Build history of the part. All positions in model axes, mm. A direction names the side the tool comes from. Give positions to 0.01 mm unless a question says otherwise; leave off trailing zeros. Order: outer loops, then holes, each group sorted by start corner. A loop starts at its lowest first (then second) coordinate and runs counter-clockwise, first axis right, second up. Notation, with made-up numbers: (-29.75, 66) - (-22.75, 66) arc R38 ccw to (-22.75, 105) - close; hole circle Ø11 at (-29, -18). An arc over 180 degrees is marked (long way). Write each question's results on one line, items separated by ' | '. Start each with the question number.
from build123d import *

# Parameters (mm, degrees)
SKETCH1_W                  = 127.078191072
SKETCH1_H                  = 113.282646321
BOSS_EXTRUDE1_DEPTH        = 39.624
SHELL_1_T                  = -2.54
OFFICIAL_RIB_BLOCK20_START = -2.54
OFFICIAL_RIB_BLOCK20_DEPTH = 2.54


with BuildPart() as part:
    # Sketch1 → Boss-Extrude1 (new body)
    with BuildSketch(Plane(origin=(0, 0, 0), x_dir=(1, 0, 0), z_dir=(0, 1, 0))):
        with Locations((1.06119575, 7.295720781)):
            Rectangle(SKETCH1_W, SKETCH1_H)
    extrude(amount=BOSS_EXTRUDE1_DEPTH)

    # 抽壳1
    shell_1_openings = [part.faces().sort_by_distance(p)[0] for p in [
        (1.06119575, 39.624, -7.295720782),
    ]]
    offset(amount=SHELL_1_T, openings=shell_1_openings, kind=Kind.INTERSECTION)

    # official_rib_block20: read off the stored shape, not the designer's step
    # official_rib_block20 outline → official_rib_block20 (add)
    with BuildSketch(Plane(origin=(0.729572078, 0, -0.729572078), x_dir=(0.7071067811865477, 0, 0.7071067811865475), z_dir=(-0.7071067811865475, 0, 0.7071067811865477)).offset(OFFICIAL_RIB_BLOCK20_START)):
        Polygon((-85.796761505, 21.08206499), (-85.796761505, 2.54), (69.764888407, 2.54), (69.764888407, 33.885045833), (7.726, 25.357), (-34.23, 35.134), align=None)
    extrude(amount=OFFICIAL_RIB_BLOCK20_DEPTH)


solid = part.part
Item 1: Which spindle directions (+Z, -Z, +X, -X, +Y, -Y) get a long thin tool onto all of the face, cutting with end or side? Do faces 1 (the flat face through (-3, 15.44, -8.05)), 2 (the flat face through (64.6, 20, -7)). Say none if no direction does.
Item 2: Cut at B-B, the plane z = -20.5. List the corners of the cut face in (x, y), then the cut area to 3 significant figures.
Item 3: Two-plate mould, pull along X, no slides. Class faces 3 (the flat face through (-62.478, 20, -7)), 4 (the flat face through (0, 0, -8)), 5 (the flat face through (15, 2.54, -20)): +X half, -X half, draft (parallel to the pull), parting line (faces both ways), or undercut.
Item 4: Flat gauge pins, fed straight in: pin 1 Ø8 at (x, z) = (8, -24) entering from +Y; pin 2 Ø10 at (x, z) = (-33, -41.5) entering from +Y. Where does each tip first touch, or does it go through?
Item 5: Probe line 1 along X through (y, z) = (33, -50); line 2 along Z through (x, y) = (23.5, 17); line 3 along X through (y, z) = (12, 40). List the from-to ranges inside material, lowest first. Write a range as from..to.
Item 6: Cut at A-A, the plane y = 8. List the corners of the cut face in (x, z).
Item 7: Cut at C-C, the plane x = -40. List the corners of the cut face in (y, z), then the cut area to 3 significant figures.
Values found:
1) face 1: +Y | face 2: +Z, -Z, +X, +Y, -Y
2) outline: (-62.48, 0) - (64.6, 0) - (64.6, 39.62) - (62.06, 39.62) - (62.06, 2.54) - (-15.45, 2.54) - (-15.45, 33.08) - (-19.04, 33.67) - (-19.04, 2.54) - (-59.94, 2.54) - (-59.94, 39.62) - (-62.48, 39.62) - close | area: 622 mm2
3) face 3: -X half | face 4: draft | face 5: undercut
4) pin 1: stops at y = 2.54 | pin 2: stops at y = 31.3
5) line 1: x = -62.48..-59.94, 62.06..64.6 | line 2: z = -63.94..-61.4, 18.45..22.04, 46.81..49.35 | line 3: x = -62.48..-59.94, 41.46..45.05, 62.06..64.6
6) outline: (-62.48, -63.94) - (64.6, -63.94) - (64.6, 49.35) - (-62.48, 49.35) - close; hole (-59.94, -61.4) - (48.26, 46.81) - (-59.94, 46.81) - close; hole (-56.35, -61.4) - (62.06, -61.4) - (62.06, 46.81) - (51.86, 46.81) - close
7) outline: (0, -63.94) - (39.62, -63.94) - (39.62, -61.4) - (2.54, -61.4) - (2.54, -45.05) - (28.07, -45.05) - (28.77, -41.46) - (2.54, -41.46) - (2.54, 46.81) - (39.62, 46.81) - (39.62, 49.35) - (0, 49.35) - close | area: 569 mm2
